Check sheet for the modelled part. Datum: model origin and axes. Units: mm. Face numbers are marked on the shaded views. A direction names the side the tool comes from. Round coordinates to 2 decimals unless told otherwise and drop trailing zeros. Write each loop counter-clockwise with the first axis right and the second up, starting at its lowest first coordinate (ties: lowest second). Pieces come first, ordered by that corner, then holes.
from build123d import *

# Parameters (mm, degrees)
F1_DEPTH  = 15
F2_R      = 2.25
F3_DEPTH  = 18
F4_R      = 2.1
F5_DEPTH  = 25
F6_W      = 3.3
F6_H      = 7
F7_DEPTH  = 25
F8_R      = 1.6
F9_SIZE   = 5
F10_DEPTH = 1.5


with BuildPart() as f1:
    # F0 (on Top) → F1 (new body)
    with BuildSketch(Plane.XY):
        Polygon((12, 0), (0, 0), (0, 16), (-3.5, 16), (-3.5, -4), (2.1, -4), (6, -4), (9.9, -4), (15.5, -4), (15.5, 16), (12, 16), align=None)
        Polygon((6, -4), (2.1, -4), (2.1, -24), (9.9, -24), (9.9, -4), align=None)
    extrude(amount=F1_DEPTH)

    # F2 (on face) → F3 (cut)
    with BuildSketch(Plane.XZ.offset(24)):
        with Locations((6, 7.5)):
            Circle(F2_R)
    extrude(amount=-F3_DEPTH, mode=Mode.SUBTRACT)

    # F4 (on face) → F5 (cut)
    with BuildSketch(Plane(origin=(-3.5, 0, 0), x_dir=(0, -1, 0), z_dir=(-1, 0, 0))):
        with Locations((-8, 7.227462)):
            Circle(F4_R)
    extrude(amount=-F5_DEPTH, mode=Mode.SUBTRACT)

    # F6 (on face) → F7 (cut)
    with BuildSketch(Plane(origin=(2.1, 0, 0), x_dir=(0, -1, 0), z_dir=(-1, 0, 0))):
        with Locations((19, 7.5)):
            Rectangle(F6_W, F6_H)
    extrude(amount=-F7_DEPTH, mode=Mode.SUBTRACT)

    # F8
    f8_edges = [f1.edges().sort_by_distance(p)[0] for p in [
        (2.1, -24, 7.5),
        (9.9, -24, 7.5),
        (-3.5, -4, 7.5),
        (15.5, -4, 7.5),
    ]]
    fillet(f8_edges, radius=F8_R)

    # F9
    f9_edges = [f1.edges().sort_by_distance(p)[0] for p in [
        (-1.75, 16, 0),
        (13.75, 16, 0),
        (13.75, 16, 15),
        (-1.75, 16, 15),
    ]]
    chamfer(f9_edges, length=F9_SIZE)

    # F4 (on face) → F10 (cut)
    with BuildSketch(Plane(origin=(-3.5, 0, 0), x_dir=(0, -1, 0), z_dir=(-1, 0, 0))):
        Polygon((-4.4, 5.149002), (-4.4, 9.305923), (-8, 11.384384), (-11.6, 9.305923), (-11.6, 5.149002), (-8, 3.070541), align=None)
        with Locations((-8, 7.227462)):
            Circle(F4_R, mode=Mode.SUBTRACT)
    extrude(amount=-F10_DEPTH, mode=Mode.SUBTRACT)


solid = f1.part
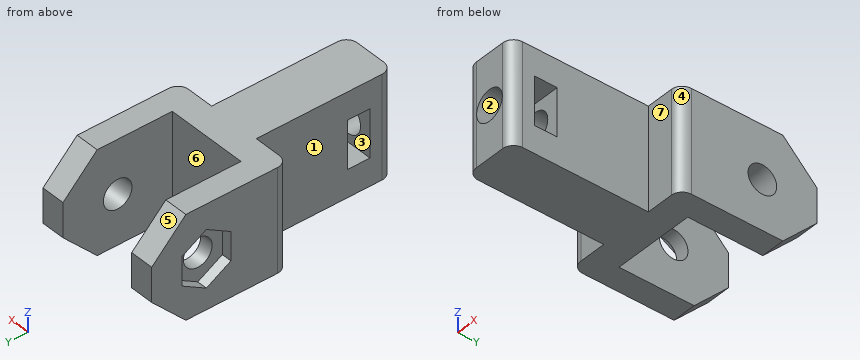
1. Release check for a two-part mould opening along X. For the marked faces 1, 2, 3 and 4 record: released by +X, released by -X, zero draft, split by the parting line, or undercut.
2. Set-up check for the marked faces 5, 6 and 7: record each of +Z, -Z, +X, -X, +Y, -Y from which the full face is reachable in a straight line by a thin tool's end or side.
3. Sectioned sample at A-A, the plane y = -19.5. Enter the section's corners in (x, z).
4. Sectioned sample at D-D, the plane x = 9.25. Enter the section's corners in (y, z).
5. Sectioned sample at C-C, the plane z = 12.75. Enter the section's corners in (x, y).
6. Sectioned sample at B-B, the plane x = 6. Enter the section's corners in (y, z), plus the area to 3 significant figures.
7. Scan lines: line 1 along X through (y, z) = (12, 1.75); line 2 along Z through (x, y) = (14.3, 8); line 3 along Z through (x, y) = (6, -14). Record each from-to range of solid material in increasing order.
8. Go/stop test with flat-tipped pins: pin 1 (6 mm diameter, centred on y = 9, z = 7, fed in from -X); pin 2 (7 mm diameter, centred on x = 6, z = 7.5, fed in from +Y); pin 3 (4.5 mm diameter, centred on y = -17.5, z = 9, fed in from +X); pin 4 (5 mm diameter, centred on x = -1.5, y = -14, fed in from +Z). Record where each tip stops, or that it passes through.
Computed values:
1. face 1: released by -X
1. face 2: undercut
1. face 3: zero draft
1. face 4: released by +X
2. face 5: +Z, +X, -X, +Y
2. face 6: +Z, -Z, +Y
2. face 7: +Z, -Z, +X, -Y
3. outline: (2.1, 0) - (9.9, 0) - (9.9, 4) - (2.1, 4) - close; (2.1, 11) - (9.9, 11) - (9.9, 15) - (2.1, 15) - close
4. outline: (-23.69, 0) - (0, 0) - (0, 15) - (-23.69, 15) - close; hole (-20.65, 4) - (-17.35, 4) - (-17.35, 11) - (-20.65, 11) - close
5. outline: (-3.5, -2.4) arc R1.6 ccw to (-1.9, -4) - (2.1, -4) - (2.1, -22.4) arc R1.6 ccw to (3.7, -24) - (8.3, -24) arc R1.6 ccw to (9.9, -22.4) - (9.9, -4) - (13.9, -4) arc R1.6 ccw to (15.5, -2.4) - (15.5, 13.25) - (12, 13.25) - (12, 0) - (0, 0) - (0, 13.25) - (-3.5, 13.25) - close
6. outline: (-24, 0) - (0, 0) - (0, 15) - (-24, 15) - (-24, 9.75) - (-20.65, 9.75) - (-20.65, 11) - (-17.35, 11) - (-17.35, 9.75) - (-6, 9.75) - (-6, 5.25) - (-17.35, 5.25) - (-17.35, 4) - (-20.65, 4) - (-20.65, 5.25) - (-24, 5.25) - close
6. area: 271 mm2
7. line 1: x = -3.5 to 0, 12 to 15.5
7. line 2: z = 0 to 5.13, 9.33 to 15
7. line 3: z = 0 to 5.25, 9.75 to 15
8. pin 1: stops at x = -3.5
8. pin 2: stops at y = 0
8. pin 3: stops at x = 9.9
8. pin 4: passes through
